The model under review builds one solid part; all positions refer to its coordinate system, in mm. Face numbers are marked on the shaded views. Round coordinates to 2 decimals unless told otherwise and drop trailing zeros. Order: outer loops, then holes, each group sorted by start corner. A loop starts at its lowest first (then second) coordinate and runs counter-clockwise, first axis right, second up. Notation, with made-up numbers: M 2.25,57 L 52.25,57 A37 ccw 52.25,94 Z; hole C 13.25,56.5 d5. An arc over 180 degrees is marked long. Use a Markdown table: item, result. Add a question column.
1. Consider section B-B on y = 1. Count the separate pieces of the cut face and the enclosed holes in it, then the cut area to 3 significant figures.
2. Insertion check: P1, Ø4, axis at x = 8, z = -6, coming from the -Y side; P2, Ø6, axis at x = 0, z = -17.68, coming from the +Y side. Each pin has a flat end and moves straight along its axis. Give the tip position at first contact, or say it passes through.
3. Consider section C-C on z = -20. State the section outline as (x, y) points.
4. Consider section A-A on x = 0. State the section outline as (y, z) points.
5. To check wall thickness, follow probe 1 along Z at (x, y) = (14, 4); probe 2 along X at (y, z) = (5.25, -1); probe 3 along X at (y, z) = (5.75, 17). State the ranges of each line that lie inside material, in increasing order.
6. The part is to be moulded in two halves that separate along X. For the marked faces 1, 2 and 3, say which applies: +X half, -X half, draft (parallel to the pull), parting line (faces both ways), or undercut.
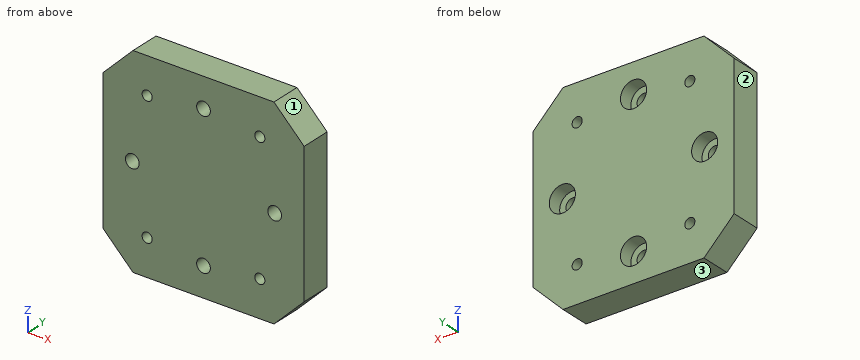
from build123d import *

# Parameters (mm, degrees)
SKETCH1_W                                           = 50
SKETCH1_H                                           = 50
BOSS_EXTRUDE1_DEPTH                                 = 7.5
M3_TAPPED_HOLE1_D                                   = 2.5
M3_TAPPED_HOLE1_DEPTH                               = 7.5
CBORE_FOR_M3_HEX_SOCKET_HEAD_CAP_SCREW1_D           = 3.4
CBORE_FOR_M3_HEX_SOCKET_HEAD_CAP_SCREW1_DEPTH       = 7.5
CBORE_FOR_M3_HEX_SOCKET_HEAD_CAP_SCREW1_CBORE_D     = 6.5
CBORE_FOR_M3_HEX_SOCKET_HEAD_CAP_SCREW1_CBORE_DEPTH = 3.4
CHAMFER1_SIZE                                       = 7.5


with BuildPart() as part:
    # Sketch1 → Boss-Extrude1 (new body)
    with BuildSketch(Plane(origin=(0, 0, 0), x_dir=(1, 0, 0), z_dir=(0, 1, 0))):
        Rectangle(SKETCH1_W, SKETCH1_H)
    extrude(amount=BOSS_EXTRUDE1_DEPTH)

    # M3 Tapped Hole1
    with Locations(Plane(origin=(0, 7.5, 0), x_dir=(1, 0, 0), z_dir=(0, 1, 0))):
        with Locations((-14, -16), (-14, 16), (14, 16), (14, -16)):
            Hole(M3_TAPPED_HOLE1_D / 2, depth=M3_TAPPED_HOLE1_DEPTH)

    # CBORE for M3 Hex Socket Head Cap Screw1
    with Locations(Plane(origin=(0, 7.5, 0), x_dir=(1, 0, 0), z_dir=(0, 1, 0))):
        with Locations((0, 17.67766953), (-17.67766953, 0), (17.67766953, 0), (0, -17.67766953)):
            CounterBoreHole(CBORE_FOR_M3_HEX_SOCKET_HEAD_CAP_SCREW1_D / 2, CBORE_FOR_M3_HEX_SOCKET_HEAD_CAP_SCREW1_CBORE_D / 2, CBORE_FOR_M3_HEX_SOCKET_HEAD_CAP_SCREW1_CBORE_DEPTH, depth=CBORE_FOR_M3_HEX_SOCKET_HEAD_CAP_SCREW1_DEPTH)

    # Chamfer1
    chamfer1_edges = [part.edges().sort_by_distance(p)[0] for p in [
        (25, 3.75, 25),
        (-25, 3.75, 25),
        (-25, 3.75, -25),
        (25, 3.75, -25),
    ]]
    chamfer(chamfer1_edges, length=CHAMFER1_SIZE)


solid = part.part
Answer block:
| question | item | result |
|---|---|---|
| 1 | separate pieces | 1 |
| 1 | enclosed holes | 8 |
| 1 | area | 2,330 mm^2 |
| 2 | P1 | y = 0 |
| 2 | P2 | y = 4.1 |
| 3 | outline | M -22.5,0 L 22.5,0 L 22.5,7.5 L 2.27,7.5 L 2.27,4.1 L -2.27,4.1 L -2.27,7.5 L -22.5,7.5 Z |
| 4 | outline | M 0,-25 L 7.5,-25 L 7.5,-20.93 L 4.1,-20.93 L 4.1,-19.38 L 0,-19.38 Z; M 0,-15.98 L 4.1,-15.98 L 4.1,-14.43 L 7.5,-14.43 L 7.5,14.43 L 4.1,14.43 L 4.1,15.98 L 0,15.98 Z; M 0,19.38 L 4.1,19.38 L 4.1,20.93 L 7.5,20.93 L 7.5,25 L 0,25 Z |
| 5 | probe 1 | -25 to -17.25, -14.75 to 14.75, 17.25 to 25 |
| 5 | probe 2 | -25 to -20.77, -14.59 to 14.59, 20.77 to 25 |
| 5 | probe 3 | -25 to -14.75, -13.25 to -3.18, 3.18 to 13.25, 14.75 to 25 |
| 6 | face 1 | +X half |
| 6 | face 2 | -X half |
| 6 | face 3 | draft |
